Work out the finished part from the listing and answer in its coordinate system (mm). A direction names the side the tool comes from. Round coordinates to 2 decimals unless told otherwise and drop trailing zeros. Write each loop counter-clockwise with the first axis right and the second up, starting at its lowest first coordinate (ties: lowest second). Pieces come first, ordered by that corner, then holes. Notation, with made-up numbers: M 40.5,-27.5 L 93.5,-27.5 A20 ccw 93.5,-7.5 Z; hole C 25.25,-15.75 d11. An arc over 180 degrees is marked long. One line per item, written item: value. Start each with the question number.
Q1. Find section D-D (y = 10). Write down the section's boundary in (x, z).
Q2. Find section A-A (y = 0). Write down the section's boundary in (x, z), and give its area (3 significant figures).
Q3. Find section C-C (z = 5). Write down the section's boundary in (x, y), and give its area (3 significant figures).
Q4. A tool of negligible diameter and unlimited length cuts with its end or side. For faces 4 (the cylindrical face through (-15.494, -4.189, 4.521)), 5 (the cylindrical face through (-16.44, 11.58, 5.07)), from which of +Z, -Z, +X, -X, +Y, -Y can it reach the whole face along a straight path? Write none if from no direction.
Q5. The mould has two halves that part along Y. Classify faces 1 (the flat face through (20.048, -7, 5)), 2 (the cylindrical face through (7.123, -11.172, 4.93)), 3 (the cylindrical face through (16.63, 11.39, 5.07)): released by +Y, released by -Y, zero draft, split by the parting line, or undercut.
Q6. Given pin 1 Ø1.2 at (x, z) = (17, 5) entering from -Y; pin 2 Ø4 at (x, y) = (5.5, 9.5) entering from +Z, each flat-ended and moving along its own axis, determine where each tip first touches the part or whether it passes through.
Q7. Find section B-B (x = 0). Write down the section's boundary in (y, z).
Q8. Consider probe 1 along Y at (x, z) = (0, 5.5); probe 2 along X at (y, z) = (-2.5, 5.5); probe 3 along Y at (x, z) = (8, 6). Determine where each line is inside the solid, lowest interval first.
Autodesk Inventor part; units mm, degrees
ref_plane "YZ Plane" through (0, 0, 0) normal (1, 0, 0) x (0, 1, 0)
ref_plane "XZ Plane" through (0, 0, 0) normal (0, 1, 0) x (-1, 0, 0)
ref_plane "XY Plane" through (0, 0, 0) normal (0, 0, 1) x (1, 0, 0)
sketch "Sketch1" plane through (0, 0, 0) normal (0, 0, 1) x (1, 0, 0)
  line L0 (16, -17.5) -> (16, 15)
  line L1 (-16, 15) -> (-16, -17.5)
  circle A0 centre (0, 0) radius 13.25
  line L2 (16, -17.5) -> (-16, -17.5)
  line L3 (-16, -17.5) -> (-16, 15)
  line L4 (16, 15) -> (-16, 15)
  dimension "d2" = 26.5
  dimension "d4" = 17.5
  dimension "d5" = 32.5
extrude "Extrusion1" add sketch "Sketch1" along normal blind 10
sketch "Sketch2" plane through (0, 0, 0) normal (0, 0, -1) x (-1, 0, 0)
  point P0 (0, 0)
sketch "Sketch3" plane through (0, 0, 0) normal (0, 0, -1) x (-1, 0, 0)
  line L0 (16, 15) -> (16, -17.5)
  line L1 (17.8498, -17.5) -> (20.048, -17.5)
  line L2 (20.048, -17.5) -> (20.048, 15)
  line L3 (20.048, 15) -> (16, 15)
  line L4 (-16, 15) -> (16, 15)
  line L5 (16, -17.5) -> (16, 15)
  line L6 (0, 0) -> (0, 7.3422)
  line L7 (-16, 15) -> (-16, -17.5)
  line L8 (-17.8498, -17.5) -> (-20.048, -17.5)
  line L9 (-20.048, -17.5) -> (-20.048, 15)
  line L10 (-20.048, 15) -> (-16, 15)
  line L11 (17.8498, -17.5) -> (16, -17.5)
  line L12 (16, 15) -> (16, -17.5)
  line L13 (20.048, 15) -> (16, 15)
  line L14 (16, -17.5) -> (-16, -17.5)
  line L15 (-17.8498, -17.5) -> (-16, -17.5)
extrude "Extrusion2" add sketch "Sketch3" against normal up to surface (10 mm away) contours L3 L2 L1 L11 L0 | L7 L15 L8 L9 L10
sketch "Sketch4" plane through (-20.048, -17.5, 0) normal (0, -1, 0) x (1, 0, 0)
  line L0 (40.0961, 0) -> (0, 0)
  line L1 (40.0961, 10) -> (0, 10)
  circle A0 centre (3.399, 5) radius 1.25
  circle A1 centre (36.697, 5) radius 1.25
  point P0 (20.048, 0)
  dimension "d11" = 2.5
extrude "Extrusion3" cut sketch "Sketch4" against normal blind 27
fillet "Fillet1" radius 12 2 edges at (20.048, 15, 5) (-20.048, 15, 5)
sketch "Sketch5" plane through (-20.048, -17.5, 0) normal (0, -1, 0) x (1, 0, 0)
  circle A0 centre (3.399, 5) radius 1.25
  circle A1 centre (36.697, 5) radius 1.25
  point P0 (20.048, 0)
  dimension "d15" = 33.298
properties part number "motor holder"
The answers:
1. outline: M -17.79,0 L -8.69,0 L -8.69,10 L -17.79,10 Z; M 8.69,0 L 17.79,0 L 17.79,10 L 8.69,10 Z
2. outline: M -20.05,0 L -13.25,0 L -13.25,10 L -20.05,10 Z; M 13.25,0 L 20.05,0 L 20.05,10 L 13.25,10 Z; hole C -16.65,5 d2.5; hole C 16.65,5 d2.5
2. area: 126 mm2
3. outline: M -20.05,-17.5 L -17.9,-17.5 L -17.9,9.5 L -15.4,9.5 L -15.4,-17.5 L 15.4,-17.5 L 15.4,9.5 L 17.9,9.5 L 17.9,-17.5 L 20.05,-17.5 L 20.05,3 A12 ccw 8.05,15 L -8.05,15 A12 ccw -20.05,3 Z; hole C 0,0 d26.5
3. area: 555 mm2
4. face 4: -Y
4. face 5: +Z, -Z, -X, +Y
5. face 1: zero draft
5. face 2: undercut
5. face 3: released by +Y
6. pin 1: y = 9.5
6. pin 2: through
7. outline: M -17.5,0 L -13.25,0 L -13.25,10 L -17.5,10 Z; M 13.25,0 L 15,0 L 15,10 L 13.25,10 Z
8. probe 1: -17.5 to -13.25, 13.25 to 15
8. probe 2: -20.05 to -17.79, -15.5 to -13.01, 13.01 to 15.5, 17.79 to 20.05
8. probe 3: -17.5 to -10.56, 10.56 to 15
